Autodesk Inventor part; units mm, degrees
ref_plane "Work Plane1" through (0, 0, 60) normal (0, 0, 1) x (1, 0, 0)
ref_plane "YZ Plane" through (0, 0, 0) normal (1, 0, 0) x (0, 1, 0)
ref_plane "XZ Plane" through (0, 0, 0) normal (0, 1, 0) x (-1, 0, 0)
sketch "Sketch1" plane through (0, 0, 0) normal (0, 0, 1) x (1, 0, 0)
  circle A0 centre (0, 0) radius 2.5
  circle A1 centre (0, 0) radius 5
  dimension "d12" = 5
  dimension "d18" = 10
sketch "Sketch3" plane through (0, 0, 0) normal (0, 0, 1) x (1, 0, 0)
  circle A0 centre (0, 0) radius 2.5
  circle A1 centre (0, 0) radius 3.75
  dimension "d14" = 5
  dimension "d15" = 7.5
extrude "Extrusion3" add sketch "Sketch3" along normal blind 90 contours A0
extrude "Extrusion4" add sketch "Sketch1" against normal blind 3.5 contours A0 | A1
thread "Thread2"
ref_plane "Work Plane1" through (0, 0, 60) normal (0, 0, 1) x (1, 0, 0)
sketch "Sketch4" plane through (0, 0, 60) normal (0, 0, 1) x (1, 0, 0)
  line L0 (-3.2481, 1.8864) -> (0.0096, 3.7562)
  line L1 (0.0096, 3.7562) -> (3.2578, 1.8698)
  line L2 (3.2578, 1.8698) -> (3.2481, -1.8864)
  line L3 (3.2481, -1.8864) -> (-0.0096, -3.7562)
  line L4 (-0.0096, -3.7562) -> (-3.2578, -1.8698)
  line L5 (-3.2578, -1.8698) -> (-3.2481, 1.8864)
  point P0 (0, 0)
  point P1 (0, 0)
extrude "Extrusion5" add sketch "Sketch4" against normal blind 4
properties part number "tornillo M5 largo"
Here's how the part is built. I have some questions about the finished solid (model axes, mm). A direction names the side the tool comes from. Coordinates: 2 decimals unless noted, no trailing zeros. Write each loop counter-clockwise with the first axis right and the second up, starting at its lowest first coordinate (ties: lowest second). Pieces come first, ordered by that corner, then holes. Notation, with made-up numbers: M 8.25,-17 L 26.25,-17 A19 cw 26.25,9 Z; hole C 39.25,-20.5 d1. An arc over 180 degrees is marked long. Answer as CSV lines item,"result". Start each with the question number.
Q1. Suppose I cut it at C-C, the plane y = 0. List the corners of the cut face in (x, z) for me, then the cut area to 3 significant figures.
Q2. If we mould it in two halves opening along Z, with no side actions, what happens to faces 5 (the flat face through (0, 3, 60)), 6 (the cylindrical face through (-0.54, 2.44, 74.79)), 7 (the flat face through (0, 0, -3.5)), 8 (the flat face through (0, 3, 56))? For each: pulls with the +Z half, pulls with the -Z half, needs draft (parallel to the pull), parting line crosses it, or undercut.
Q3. I need wall thicknesses on probe 1 along Z at (x, y) = (1, 2.5); probe 2 along Z at (x, y) = (4, 0.25); probe 3 along X at (y, z) = (-0.25, 36.5). Which ranges of each line are inside material? Lowest first, please. Write a range as [from, to].
Q4. Will these pins go through, and if not, where does the flat tip stop? pin 1 Ø1 at (x, z) = (2.5, 16) entering from +Y; pin 2 Ø2 at (y, z) = (-4, 57) entering from +X; pin 3 Ø5 at (x, y) = (1, 4) entering from +Z; pin 4 Ø6 at (y, z) = (-1, 19.5) entering from +X.
Q5. Suppose I cut it at B-B, the plane z = 68.5. List the corners of the cut face in (x, y) for me, then the cut area to 3 significant figures.
Q6. Suppose I cut it at A-A, the plane x = 1.5. List the corners of the cut face in (y, z) for me.
Q7. For faces 1 (the cylindrical face through (-0.54, 2.44, 27.61)), 2 (the flat face through (-1.611, -2.826, 58.028)), 3 (the flat face through (1.611, 2.826, 58.028)), 4 (the flat face through (1.64, -2.81, 58.03)), which set-ups out of +Z, -Z, +X, -X, +Y, -Y let a thin tool reach every point of the face, with its end or its side?
Entries:
1,outline,"M -5,-3.5 L 5,-3.5 L 5,0 L 2.5,0 L 2.5,56 L 3.25,56 L 3.25,60 L 2.5,60 L 2.5,90 L -2.5,90 L -2.5,60 L -3.25,60 L -3.25,56 L -2.5,56 L -2.5,0 L -5,0 Z"
1,area,"491 mm²"
2,face 5,"pulls with the +Z half"
2,face 6,"needs draft"
2,face 7,"pulls with the -Z half"
2,face 8,"undercut"
3,probe 1,"z = [-3.5, 0], [56, 60]"
3,probe 2,"z = [-3.5, 0]"
3,probe 3,"x = [-2.49, 2.49]"
4,pin 1,"stops at y = 1.5"
4,pin 2,"stops at x = 1.31"
4,pin 3,"stops at z = 90"
4,pin 4,"stops at x = 2.5"
5,outline,"C 0,0 d5"
5,area,"19.6 mm²"
6,outline,"M -4.77,-3.5 L 4.77,-3.5 L 4.77,0 L 2,0 L 2,56 L 2.89,56 L 2.89,60 L 2,60 L 2,90 L -2,90 L -2,60 L -2.89,60 L -2.89,56 L -2,56 L -2,0 L -4.77,0 Z"
7,face 1,"none"
7,face 2,"+Z, -X, -Y"
7,face 3,"+Z, +X, +Y"
7,face 4,"+Z, +X, -Y"
